Verification items for the finished model (mm, model axes). A direction names the side the tool comes from. Coordinates: 2 decimals unless noted, no trailing zeros. Write each loop counter-clockwise with the first axis right and the second up, starting at its lowest first coordinate (ties: lowest second). Pieces come first, ordered by that corner, then holes. Notation, with made-up numbers: (1.5, -26.5) -> (16.5, -26.5) arc R13 ccw to (16.5, -19.5) -> close; hole circle Ø7 at (71.5, 36.25). An arc over 180 degrees is marked (long way). Write item = value, one per line. Start each with the question number.
(1) Section check A-A (z = 8). Record the cut outline in (x, y).
(2) Set-up check for faces 1 (the face through (7.9, -3.04, 25.04)), 2 (the face through (8.45, -2, 9)), 3 (the face through (-15.075, 0, 1)): record each of +Z, -Z, +X, -X, +Y, -Y from which the full face is reachable in a straight line by a thin tool's end or side.
(3) Material ranges on probe 1 along X at (y, z) = (-0.5, 7.25); probe 2 along X at (y, z) = (0, 4.45); probe 3 along X at (y, z) = (-6.5, 20), recorded low to high. Write a range as [from, to].
(4) Gauge pin test, flat ends, axial feed: pin 1 Ø1.5 at (y, z) = (1.5, 16) entering from -X; pin 2 Ø4 at (y, z) = (-2.45, 23.45) entering from -X; pin 3 Ø2 at (x, y) = (5, -5) entering from +Z; pin 4 Ø1 at (x, y) = (15, 1.5) entering from -Z. Record the tip position at first contact, or that the pin passes through.
(5) Section check C-C (z = 21). Record the cut outline in (x, y), plus the area to 3 significant figures.
(6) Mould release check, pull along Y, two halves, no side actions. Record for faces 4 (the face through (0, 9.45, 12)), 5 (the face through (1.05, 2, 9)), 6 (the face through (6.9, -3.04, 25.04)): released by +Y, released by -Y, zero draft, split by the parting line, or undercut.
(7) Section check D-D (x = 19.9). Record the cut outline in (y, z), plus the area to 3 significant figures.
(8) Section check B-B (z = 3). State how many separate pieces and enclosed holes the cut face has, plus the area to 3 significant figures.
```python
from build123d import *

# Parameters (mm, degrees)
BOSS_EXTRUDE1_DEPTH = 1.65
SKETCH2_R           = 1.650000009
BOSS_EXTRUDE2_DEPTH = 4
BOSS_EXTRUDE3_DEPTH = 13
CUT_EXTRUDE1_DEPTH  = 16.5
FILLET1_R           = 4
FILLET2_R           = 3
SKETCH5_R           = 2.5
CUT_EXTRUDE2_DEPTH  = 1.9
SKETCH6_W           = 5.2
SKETCH6_H           = 10.2
BOSS_EXTRUDE4_DEPTH = 1.6
FILLET3_R           = 1
SKETCH7_W           = 2.1
SKETCH7_H           = 4
BOSS_EXTRUDE5_DEPTH = 15.2
FILLET4_R           = 1
SKETCH8_W           = 1
SKETCH8_H           = 5
BOSS_EXTRUDE6_DEPTH = 6.7
SKETCH9_R           = 1.5
CUT_EXTRUDE3_DEPTH  = 44.75417123
CUT_EXTRUDE4_REACH  = 40.548
SKETCH10_R          = 1.5


with BuildPart() as part:
    # Sketch1 → Boss-Extrude1 (new body)
    with BuildSketch(Plane.XY):
        with BuildLine():
            Line((-13.075, -11.05), (13.075, -11.05))
            ThreePointArc((13.075, -11.05), (14.489213562, -10.464213562), (15.075, -9.05))
            Line((15.075, -9.05), (15.075, 9.05))
            ThreePointArc((15.075, 9.05), (14.489213562, 10.464213562), (13.075, 11.05))
            Line((13.075, 11.05), (-13.075, 11.05))
            ThreePointArc((-13.075, 11.05), (-14.489213562, 10.464213562), (-15.075, 9.05))
            Line((-15.075, 9.05), (-15.075, -9.05))
            ThreePointArc((-15.075, -9.05), (-14.489213562, -10.464213562), (-13.075, -11.05))
        make_face()
    extrude(amount=BOSS_EXTRUDE1_DEPTH)

    # Sketch2 → Boss-Extrude2 (add)
    with BuildSketch(Plane.XY.offset(1.65)):
        with BuildLine():
            Line((14.317737301, 10.617036694), (22.913637955, 3.800063983))
            ThreePointArc((22.913637955, 3.800063983), (24.75, 0), (22.913637955, -3.800063983))
            Line((22.913637955, -3.800063983), (14.317737301, -10.617036694))
            ThreePointArc((14.317737301, -10.617036694), (13.732999473, -10.938660026), (13.075, -11.05))
            Line((13.075, -11.05), (-13.075, -11.05))
            ThreePointArc((-13.075, -11.05), (-13.732999473, -10.938660026), (-14.317737301, -10.617036694))
            Line((-14.317737301, -10.617036694), (-22.913637955, -3.800063983))
            ThreePointArc((-22.913637955, -3.800063983), (-24.75, 0), (-22.913637955, 3.800063983))
            Line((-22.913637955, 3.800063983), (-14.317737301, 10.617036694))
            ThreePointArc((-14.317737301, 10.617036694), (-13.732999473, 10.938660026), (-13.075, 11.05))
            Line((-13.075, 11.05), (13.075, 11.05))
            ThreePointArc((13.075, 11.05), (13.732999473, 10.938660026), (14.317737301, 10.617036694))
        make_face()
        with Locations((19.9, 0)):
            Circle(SKETCH2_R, mode=Mode.SUBTRACT)
        with Locations((-19.9, 0)):
            Circle(SKETCH2_R, mode=Mode.SUBTRACT)
    extrude(amount=BOSS_EXTRUDE2_DEPTH)

    # Sketch3 → Boss-Extrude3 (add)
    with BuildSketch(Plane.XY.offset(5.65)):
        Polygon((-8.5, 9.45), (8.5, 9.45), (13.5, 4.2), (13.5, -9.35), (-13.5, -9.35), (-13.5, 4.2), align=None)
    extrude(amount=BOSS_EXTRUDE3_DEPTH)

    # Sketch4 → Cut-Extrude1 (cut)
    with BuildSketch(Plane(origin=(0, 0, 0), x_dir=(-1, 0, 0), z_dir=(0, 0, -1))):
        Polygon((-8.35, 7.95), (8.35, 7.95), (12, 4.55), (12, -7.65), (-12, -7.65), (-12, 4.55), align=None)
    extrude(amount=-CUT_EXTRUDE1_DEPTH, mode=Mode.SUBTRACT)

    # Fillet1
    fillet1_edges = [part.edges().sort_by_distance(p)[0] for p in [
        (-13.5, -9.35, 12.15),
        (13.5, -9.35, 12.15),
    ]]
    fillet(fillet1_edges, radius=FILLET1_R)

    # Fillet2
    fillet2_edges = [part.edges().sort_by_distance(p)[0] for p in [
        (-12, -7.65, 8.25),
        (12, -7.65, 8.25),
    ]]
    fillet(fillet2_edges, radius=FILLET2_R)

    # Sketch5 → Cut-Extrude2 (cut)
    with BuildSketch(Plane(origin=(0, 0, 1.65), x_dir=(-1, 0, 0), z_dir=(0, 0, -1))):
        with Locations((-19.9, 0)):
            Circle(SKETCH5_R)
        with Locations((19.9, 0)):
            Circle(SKETCH5_R)
    extrude(amount=-CUT_EXTRUDE2_DEPTH, mode=Mode.SUBTRACT)

    # Sketch6 → Boss-Extrude4 (add)
    with BuildSketch(Plane.XY.offset(18.65)):
        with Locations((0, 3.65)):
            Rectangle(SKETCH6_W, SKETCH6_H)
        with Locations((7.4, -3.65)):
            Rectangle(SKETCH6_W, SKETCH6_H)
        with Locations((-7.4, -3.65)):
            Rectangle(SKETCH6_W, SKETCH6_H)
    extrude(amount=BOSS_EXTRUDE4_DEPTH)

    # Fillet3
    fillet3_edges = [part.edges().sort_by_distance(p)[0] for p in [
        (-2.6, 8.75, 19.45),
        (-2.6, -1.45, 19.45),
        (2.6, -1.45, 19.45),
        (2.6, 8.75, 19.45),
        (4.8, 1.45, 19.45),
        (4.8, -8.75, 19.45),
        (10, -8.75, 19.45),
        (10, 1.45, 19.45),
        (-10, 1.45, 19.45),
        (-10, -8.75, 19.45),
        (-4.8, -8.75, 19.45),
        (-4.8, 1.45, 19.45),
    ]]
    fillet(fillet3_edges, radius=FILLET3_R)

    # Sketch7 → Boss-Extrude5 (add)
    with BuildSketch(Plane(origin=(0, 0, 16.5), x_dir=(-1, 0, 0), z_dir=(0, 0, -1))):
        with Locations((0, 2.05)):
            Rectangle(SKETCH7_W, SKETCH7_H)
        with Locations((-7.4, -2.05)):
            Rectangle(SKETCH7_W, SKETCH7_H)
        with Locations((7.4, -2.05)):
            Rectangle(SKETCH7_W, SKETCH7_H)
    extrude(amount=BOSS_EXTRUDE5_DEPTH)

    # Fillet4
    fillet4_edges = [part.edges().sort_by_distance(p)[0] for p in [
        (1.05, 2.05, 1.3),
        (-1.05, 2.05, 1.3),
        (8.45, -2.05, 1.3),
        (6.35, -2.05, 1.3),
        (-6.35, -2.05, 1.3),
        (-8.45, -2.05, 1.3),
    ]]
    fillet(fillet4_edges, radius=FILLET4_R)

    # Sketch8 → Boss-Extrude6 (add)
    with BuildSketch(Plane.XY.offset(20.25)):
        with Locations((-7.4, -2.45)):
            Rectangle(SKETCH8_W, SKETCH8_H)
        with Locations((0, 2.55)):
            Rectangle(SKETCH8_W, SKETCH8_H)
        with Locations((7.4, -2.45)):
            Rectangle(SKETCH8_W, SKETCH8_H)
    extrude(amount=BOSS_EXTRUDE6_DEPTH)

    # Sketch9 → Cut-Extrude3 (cut, through all)
    with BuildSketch(Plane.ZY.offset(7.9)):
        with Locations((23.45, -2.45)):
            Circle(SKETCH9_R)
        Polygon((25.797828138, 0.05), (26.95, -1.2), (26.95, 0.05), align=None)
        Polygon((26.95, -3.7), (25.797828138, -4.95), (26.95, -4.95), align=None)
    extrude(amount=-CUT_EXTRUDE3_DEPTH, mode=Mode.SUBTRACT)

    # Sketch10 → Cut-Extrude4 (cut, up to next)
    with BuildSketch(Plane.ZY.offset(0.5), mode=Mode.PRIVATE) as cut_extrude4_sk1:
        with Locations((23.95, 2.55)):
            Circle(SKETCH10_R)
    cut_extrude4_tool1 = extrude(cut_extrude4_sk1.sketch, amount=-CUT_EXTRUDE4_REACH, mode=Mode.PRIVATE) & part.part
    # Sketch10 → Cut-Extrude4 (cut, up to next)
    with BuildSketch(Plane.ZY.offset(0.5), mode=Mode.PRIVATE) as cut_extrude4_sk2:
        Polygon((25.3887505, 5.05), (26.95, 3.8), (26.95, 5.05), align=None)
    cut_extrude4_tool2 = extrude(cut_extrude4_sk2.sketch, amount=-CUT_EXTRUDE4_REACH, mode=Mode.PRIVATE) & part.part
    # Sketch10 → Cut-Extrude4 (cut, up to next)
    with BuildSketch(Plane.ZY.offset(0.5), mode=Mode.PRIVATE) as cut_extrude4_sk3:
        Polygon((26.95, 1.3), (25.3887505, 0.05), (26.95, 0.05), align=None)
    cut_extrude4_tool3 = extrude(cut_extrude4_sk3.sketch, amount=-CUT_EXTRUDE4_REACH, mode=Mode.PRIVATE) & part.part
    add(cut_extrude4_tool1.solids().sort_by_distance((-0.5, 2.55, 23.95))[0], mode=Mode.SUBTRACT)
    add(cut_extrude4_tool2.solids().sort_by_distance((-0.5, 4.633333, 26.429584))[0], mode=Mode.SUBTRACT)
    add(cut_extrude4_tool3.solids().sort_by_distance((-0.5, 0.466667, 26.429584))[0], mode=Mode.SUBTRACT)


solid = part.part
```
Response:
q1.outline = (-13.5, -5.35) arc R4 ccw to (-9.5, -9.35) -> (9.5, -9.35) arc R4 ccw to (13.5, -5.35) -> (13.5, 4.2) -> (8.5, 9.45) -> (-8.5, 9.45) -> (-13.5, 4.2) -> close; (-8.45, -4.05) -> (-6.35, -4.05) -> (-6.35, -0.05) -> (-8.45, -0.05) -> close; (-1.05, 0.05) -> (1.05, 0.05) -> (1.05, 4.05) -> (-1.05, 4.05) -> close; (6.35, -4.05) -> (8.45, -4.05) -> (8.45, -0.05) -> (6.35, -0.05) -> close; hole (-12, -4.65) arc R3 ccw to (-9, -7.65) -> (9, -7.65) arc R3 ccw to (12, -4.65) -> (12, 4.55) -> (8.35, 7.95) -> (-8.35, 7.95) -> (-12, 4.55) -> close
q2.face_1 = +Z, +X, +Y, -Y
q2.face_2 = -Z
q2.face_3 = -Z, -X, +Y, -Y
q3.probe_1 = [-13.5, -12], [-8.45, -6.35], [6.35, 8.45], [12, 13.5]
q3.probe_2 = [-24.75, -21.55], [-18.25, -12], [12, 18.25], [21.55, 24.75]
q3.probe_3 = [-10, -4.8], [4.8, 10]
q4.pin_1 = -13.5
q4.pin_2 = -7.9
q4.pin_3 = 20.25
q4.pin_4 = 0
q5.outline = (-7.9, -4.95) -> (-6.9, -4.95) -> (-6.9, 0.05) -> (-7.9, 0.05) -> close; (-0.5, 0.05) -> (0.5, 0.05) -> (0.5, 5.05) -> (-0.5, 5.05) -> close; (6.9, -4.95) -> (7.9, -4.95) -> (7.9, 0.05) -> (6.9, 0.05) -> close
q5.area = 15.0 mm2
q6.face_4 = released by +Y
q6.face_5 = undercut
q6.face_6 = zero draft
q7.outline = (-6.19, 1.65) -> (-2.5, 1.65) -> (-2.5, 3.55) -> (-1.65, 3.55) -> (-1.65, 5.65) -> (-6.19, 5.65) -> close; (1.65, 3.55) -> (2.5, 3.55) -> (2.5, 1.65) -> (6.19, 1.65) -> (6.19, 5.65) -> (1.65, 5.65) -> close
q7.area = 33.1 mm2
q8.separate_pieces = 4
q8.enclosed_holes = 3
q8.area = 527 mm2
